Could you check a few things on this model? Use its own coordinates, in mm. Face numbers are marked on the shaded views. A direction names the side the tool comes from. Give positions to 0.01 mm unless a question says otherwise; leave off trailing zeros. Loops run counter-clockwise (first coordinate to the right, second up) from the corner with the lowest first, then second, coordinate; pieces in that order, holes last. Notation, with made-up numbers: (8, 24.5) -> (67, 24.5) arc R21 ccw to (67, 51.5) -> close; hole circle Ø10 at (32.25, 44.5). An arc over 180 degrees is marked (long way). Write item = value, one per line. Start each with the question number.
1) On a 3-axis mill with a long thin cutter (end or side, diameter ignored), from which of +Z, -Z, +X, -X, +Y, -Y can I reach the whole of each face in a straight line? I mean the marked faces 1, 2, 3, 4 and 5. Say none if no direction works.
2) I want a section at A-A (z = -14). List the corners of the cut face in (x, y) for me.
3) I want a section at D-D (y = 13.5). List the corners of the cut face in (x, z) for me, and give its area (3 significant figures).
4) If we mould it in two halves opening along Y, with no side actions, what happens to the marked faces 6, 7 and 8? For each: +Y half, -Y half, draft (parallel to the pull), parting line (faces both ways), or undercut.
5) I want a section at C-C (x = 11). List the corners of the cut face in (y, z) for me, and give its area (3 significant figures).
6) I want a section at B-B (y = 0). List the corners of the cut face in (x, z) for me, and give its area (3 significant figures).
7) I need wall thicknesses on probe 1 along Z at (x, y) = (-7.25, 0); probe 2 along Z at (x, y) = (1.25, 0); probe 3 along Y at (x, z) = (-1.5, 0.5). Which ranges of each line are inside material? Lowest first, please. Write a range as from..to.
8) I'm going to push flat-ended pins straight in: pin 1 Ø1.2 at (x, y) = (3, -13) entering from +Z; pin 2 Ø4 at (x, z) = (4, 9) entering from +Y; pin 3 Ø4.5 at (x, z) = (5, -13) entering from -Y. Where does each tip first touch, or does it pass through?
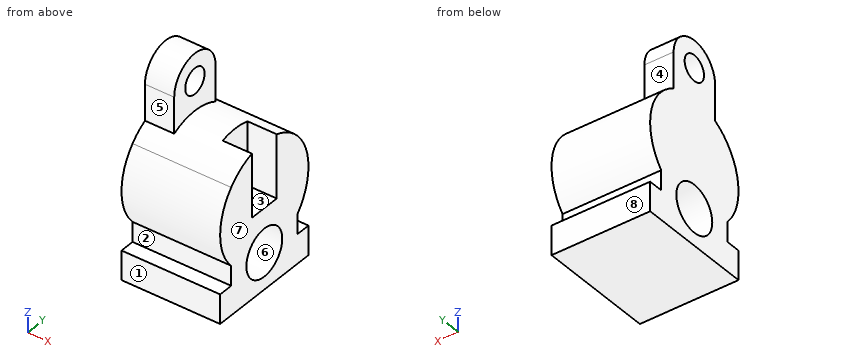
from build123d import *

# Parameters (mm, degrees)
F0_W          = 4
F0_H          = 8
F1_DEPTH      = 13.5
F3_D          = 13
F4_W          = 8
F4_H          = 9
F4_H_2        = 3
F5_DEPTH      = 31.5
F6_DEPTH      = 110
F6_DEPTH_BACK = 2
F8_D          = 7
F9_DEPTH      = 25


with BuildPart() as f1:
    # F0 (on Right) → F1 (new body, symmetric)
    with BuildSketch(Plane.YZ):
        with BuildLine():
            Line((12, 0), (12, 10.5830052443))
            ThreePointArc((12, 10.5830052443), (0, 16), (-12, 10.5830052443))
            Line((-12, 10.5830052443), (-12, 0))
            Line((-12, 0), (12, 0))
        make_face()
        with BuildLine():
            Line((12, 0), (16, 0))
            ThreePointArc((16, 0), (14.9666295471, 5.6568542495), (12, 10.5830052443))
            Line((12, 10.5830052443), (12, 0))
        make_face()
        with BuildLine():
            Line((12, -10.5830052443), (12, 0))
            Line((12, 0), (-12, 0))
            Line((-12, 0), (-12, -10.5830052443))
            ThreePointArc((-12, -10.5830052443), (-6.5830052443, -14.5830052443), (0, -16))
            ThreePointArc((0, -16), (6.5830052443, -14.5830052443), (12, -10.5830052443))
        make_face()
        with BuildLine():
            ThreePointArc((12, -10.5830052443), (14.9666295471, -5.6568542495), (16, 0))
            Line((16, 0), (12, 0))
            Line((12, 0), (12, -10.5830052443))
        make_face()
        with BuildLine():
            Line((-12, 0), (-12, 10.5830052443))
            ThreePointArc((-12, 10.5830052443), (-14.9666295471, 5.6568542495), (-16, 0))
            Line((-16, 0), (-12, 0))
        make_face()
        with BuildLine():
            Line((-12, -10.5830052443), (-12, 0))
            Line((-12, 0), (-16, 0))
            ThreePointArc((-16, 0), (-14.9666295471, -5.6568542495), (-12, -10.5830052443))
        make_face()
        with BuildLine():
            Line((-12, -16), (0, -16))
            ThreePointArc((0, -16), (-6.5830052443, -14.5830052443), (-12, -10.5830052443))
            Line((-12, -10.5830052443), (-12, -16))
        make_face()
        Polygon((12, -24), (12, -16), (0, -16), (-12, -16), (-12, -24), align=None)
        with Locations((-14, -20)):
            Rectangle(F0_W, F0_H)
        with BuildLine():
            Line((12, -16), (12, -10.5830052443))
            ThreePointArc((12, -10.5830052443), (6.5830052443, -14.5830052443), (0, -16))
            Line((0, -16), (12, -16))
        make_face()
        with Locations((14, -20)):
            Rectangle(F0_W, F0_H)
    extrude(amount=F1_DEPTH, both=True)

    # F3 (through all)
    with Locations(Plane.YZ.offset(13.5)):
        with Locations((0, -14)):
            Hole(F3_D / 2)

    # F4 (on Top) → F5 (join)
    with BuildSketch(Plane.XY):
        with Locations((-9.5, 0)):
            Rectangle(F4_W, F4_H)
        with Locations((-9.5, 6)):
            Rectangle(F4_W, F4_H_2)
        with Locations((-9.5, -6)):
            Rectangle(F4_W, F4_H_2)
    extrude(amount=F5_DEPTH)

    # F4 (on Top) → F6 (cut, two sides)
    with BuildSketch(Plane.XY) as f6_sk:
        with Locations((9.5, 0)):
            Rectangle(F4_W, F4_H)
    extrude(amount=F6_DEPTH, mode=Mode.SUBTRACT)
    extrude(f6_sk.sketch, amount=-F6_DEPTH_BACK, mode=Mode.SUBTRACT)

    # F8 (through all)
    with Locations(Plane(origin=(-13.5, 0, 0), x_dir=(0, -1, 0), z_dir=(-1, 0, 0))):
        with Locations((0, 24)):
            Hole(F8_D / 2)

    # F7 (on face) → F9 (cut)
    with BuildSketch(Plane(origin=(-13.5, 0, 0), x_dir=(0, -1, 0), z_dir=(-1, 0, 0))):
        with BuildLine():
            Line((7.5, 24), (7.5, 31.5))
            Line((7.5, 31.5), (0, 31.5))
            ThreePointArc((0, 31.5), (5.3033008589, 29.3033008589), (7.5, 24))
        make_face()
        with BuildLine():
            ThreePointArc((-7.5, 24), (-5.3033008589, 29.3033008589), (0, 31.5))
            Line((0, 31.5), (-7.5, 31.5))
            Line((-7.5, 31.5), (-7.5, 24))
        make_face()
    extrude(amount=-F9_DEPTH, mode=Mode.SUBTRACT)


solid = f1.part
Answer list:
q1.face_1 = +Z, -Z, +X, -X, -Y
q1.face_2 = +X, -X, -Y
q1.face_3 = +Z, +X
q1.face_4 = +Z, +X, -X, +Y
q1.face_5 = +Z, +X, -X, -Y
q2.outline = (-13.5, -12) -> (13.5, -12) -> (13.5, -6.5) -> (-13.5, -6.5) -> close; (-13.5, 6.5) -> (13.5, 6.5) -> (13.5, 12) -> (-13.5, 12) -> close
q3.outline = (-13.5, -24) -> (13.5, -24) -> (13.5, -16) -> (-13.5, -16) -> close; (-13.5, -8.59) -> (13.5, -8.59) -> (13.5, 8.59) -> (-13.5, 8.59) -> close
q3.area = 680 mm^2
q4.face_6 = undercut
q4.face_7 = draft
q4.face_8 = +Y half
q5.outline = (-16, -24) -> (16, -24) -> (16, -16) -> (12, -16) -> (12, -10.58) arc R16 ccw to (4.5, 15.35) -> (4.5, -2) -> (-4.5, -2) -> (-4.5, 15.35) arc R16 ccw to (-12, -10.58) -> (-12, -16) -> (-16, -16) -> close; hole circle Ø13 at (0, -14)
q5.area = 807 mm^2
q6.outline = (-13.5, -24) -> (13.5, -24) -> (13.5, -20.5) -> (-13.5, -20.5) -> close; (-13.5, -7.5) -> (13.5, -7.5) -> (13.5, -2) -> (5.5, -2) -> (5.5, 16) -> (-5.5, 16) -> (-5.5, 20.5) -> (-13.5, 20.5) -> close; (-13.5, 27.5) -> (-5.5, 27.5) -> (-5.5, 31.5) -> (-13.5, 31.5) -> close
q6.area = 653 mm^2
q7.probe_1 = -24..-20.5, -7.5..20.5, 27.5..31.5
q7.probe_2 = -24..-20.5, -7.5..16
q7.probe_3 = -15.99..15.99
q8.pin_1 = 10.11
q8.pin_2 = 14.39
q8.pin_3 = -12
